For this review, take the finished solid that the model builds, in its own axes (mm). Face numbers are marked on the shaded views. Round coordinates to 2 decimals unless told otherwise and drop trailing zeros. Write each loop counter-clockwise with the first axis right and the second up, starting at its lowest first coordinate (ties: lowest second). Pieces come first, ordered by that corner, then holes. Notation, with made-up numbers: (-22, -31.75) - (-4, -31.75) arc R4 ccw to (-4, -27.75) - close; hole circle Ø2 at (-34.75, 1.25). An arc over 180 degrees is marked (long way). One line per item, written item: value. Start each with the question number.
Q1. Add section C-C on z = -231. Write out the cut boundary in (x, y), and give its area (3 significant figures).
Q2. Mouldability with a two-part tool opening along Z and no side actions: class the marked faces 1, 2 and 3 as +Z half, -Z half, draft (parallel to the pull), parting line (faces both ways), or undercut.
Q3. Add section B-B on z = -33. Write out the cut boundary in (x, y), and give its area (3 significant figures).
Q4. Clearance check with flat-ended pins moving along their axes: pin 1 Ø20.5 at (x, y) = (578.5, -461.5) entering from -Z; pin 2 Ø12.5 at (x, z) = (222, -82) entering from +Y; pin 3 Ø1 at (y, z) = (-207, -108) entering from +X. State where each tip first meets the part, or that it passes through.
Q5. Add section D-D on x = 97.5. Write out the cut boundary in (y, z).
Q6. Add section A-A on y = -127. Write out the cut boundary in (x, z), and give its area (3 significant figures).
Q7. For probe 1 along X at (y, z) = (-132.5, -85); probe 2 along Z at (x, y) = (92, -295.5); probe 3 along Z at (x, y) = (464, -364), list the stretches that pass through material, from the lowest coordinate up.
```python
from build123d import *

# Parameters (mm, degrees)
CROQUIS1_W               = 491.3875
CROQUIS1_H               = 491.3875
CROQUIS1_W_2             = 440.5875
CROQUIS1_H_2             = 440.5875
SALIENTE_EXTRUIR1_DEPTH  = 25.4
CROQUIS2_W               = 25.4
CROQUIS2_H               = 25.4
SALIENTE_EXTRUIR2_DEPTH  = 422.312858808
CROQUIS3_W               = 25.4
CROQUIS3_H               = 25.4
SALIENTE_EXTRUIR3_DEPTH  = 25.4
SALIENTE_EXTRUIR4_REACH  = 813.249
CROQUIS4_W               = 25.4
CROQUIS4_H               = 25.4
CROQUIS5_W               = 25.4
CROQUIS5_H               = 25.4
SALIENTE_EXTRUIR5_DEPTH  = 292
SALIENTE_EXTRUIR7_REACH  = 813.249
CROQUIS7_W               = 25.4
CROQUIS7_H               = 25.4
SALIENTE_EXTRUIR9_DEPTH  = 25.4
SALIENTE_EXTRUIR10_DEPTH = 25.4
SALIENTE_EXTRUIR11_REACH = 950.384
CROQUIS11_W              = 25.4
CROQUIS11_H              = 25.4
SALIENTE_EXTRUIR12_DEPTH = 25.4
SALIENTE_EXTRUIR13_REACH = 932.183
CROQUIS13_W              = 25.087212933
CROQUIS13_H              = 25.4
SALIENTE_EXTRUIR8_DEPTH  = 0.79375


with BuildPart() as part:
    # Croquis1 → Saliente-Extruir1 (new body)
    with BuildSketch(Plane(origin=(0, 0, 0), x_dir=(1, 0, 0), z_dir=(0, 1, 0))):
        with Locations((220.29375, 220.29375)):
            Rectangle(CROQUIS1_W, CROQUIS1_H)
        with Locations((220.29375, 220.29375)):
            Rectangle(CROQUIS1_W_2, CROQUIS1_H_2, mode=Mode.SUBTRACT)
    extrude(amount=-SALIENTE_EXTRUIR1_DEPTH)

    # Croquis2 → Saliente-Extruir2 (add)
    with BuildSketch(Plane.XZ.offset(25.4)):
        with Locations((453.2875, -369.3875)):
            Rectangle(CROQUIS2_W, CROQUIS2_H)
        with Locations((-12.7, -369.3875)):
            Rectangle(CROQUIS2_W, CROQUIS2_H)
    extrude(amount=SALIENTE_EXTRUIR2_DEPTH)

    # Croquis3 → Saliente-Extruir3 (add)
    with BuildSketch(Plane.XZ.offset(447.712858808)):
        with Locations((-12.7, -369.3875)):
            Rectangle(CROQUIS3_W, CROQUIS3_H)
        with Locations((453.2875, -369.3875)):
            Rectangle(CROQUIS3_W, CROQUIS3_H)
    extrude(amount=SALIENTE_EXTRUIR3_DEPTH)

    # Croquis4 → Saliente-Extruir4 (add, up to next)
    with BuildSketch(Plane(origin=(0, 0, 0), x_dir=(0, 0, -1), z_dir=(1, 0, 0)), mode=Mode.PRIVATE) as saliente_extruir4_sk1:
        with Locations((369.3875, -460.412858808)):
            Rectangle(CROQUIS4_W, CROQUIS4_H)
    saliente_extruir4_tool1 = extrude(saliente_extruir4_sk1.sketch, amount=SALIENTE_EXTRUIR4_REACH, mode=Mode.PRIVATE) - part.part
    add(saliente_extruir4_tool1.solids().sort_by_distance((0, -460.412859, -369.3875))[0])

    # Croquis5 → Saliente-Extruir5 (add)
    with BuildSketch(Plane.XY.offset(-356.6875)):
        with Locations((-12.7, -460.412858808)):
            Rectangle(CROQUIS5_W, CROQUIS5_H)
        with Locations((453.2875, -460.412858808)):
            Rectangle(CROQUIS5_W, CROQUIS5_H)
    extrude(amount=SALIENTE_EXTRUIR5_DEPTH)

    # Croquis7 → Saliente-Extruir7 (add, up to next)
    with BuildSketch(Plane(origin=(0, 0, 0), x_dir=(0, 0, -1), z_dir=(1, 0, 0)), mode=Mode.PRIVATE) as saliente_extruir7_sk1:
        with Locations((369.3875, -255.012858808)):
            Rectangle(CROQUIS7_W, CROQUIS7_H)
    saliente_extruir7_tool1 = extrude(saliente_extruir7_sk1.sketch, amount=SALIENTE_EXTRUIR7_REACH, mode=Mode.PRIVATE) - part.part
    add(saliente_extruir7_tool1.solids().sort_by_distance((0, -255.012859, -369.3875))[0])

    # Croquis9 → Saliente-Extruir9 (add)
    with BuildSketch(Plane(origin=(0, -447.712858808, 0), x_dir=(1, 0, 0), z_dir=(0, 1, 0))):
        Polygon((465.9875, 382.0875), (694.147848124, 382.0875), (694.147848124, 65.242422269), (465.9875, 65.242422269), (0, 65.242422269), (0, 90.642422269), (465.9875, 90.642422269), (668.747848124, 90.642422269), (668.747848124, 356.6875), (465.9875, 356.6875), align=None)
    extrude(amount=-SALIENTE_EXTRUIR9_DEPTH)

    # Croquis10 → Saliente-Extruir10 (add)
    with BuildSketch(Plane.XY.offset(-356.6875)):
        Polygon((668.747848124, -447.712858808), (668.747848124, -267.712858808), (465.9875, -267.712858808), (465.9875, -191.947517804), (694.147848124, -242.312858808), (694.147848124, -447.712858808), align=None)
    extrude(amount=-SALIENTE_EXTRUIR10_DEPTH)

    # Croquis11 → Saliente-Extruir11 (add, up to next)
    with BuildSketch(Plane(origin=(0, -447.712858808, 0), x_dir=(1, 0, 0), z_dir=(0, 1, 0)), mode=Mode.PRIVATE) as saliente_extruir11_sk1:
        with Locations((-12.7, 77.942422269)):
            Rectangle(CROQUIS11_W, CROQUIS11_H)
    saliente_extruir11_tool1 = extrude(saliente_extruir11_sk1.sketch, amount=SALIENTE_EXTRUIR11_REACH, mode=Mode.PRIVATE) - part.part
    # Croquis11 → Saliente-Extruir11 (add, up to next)
    with BuildSketch(Plane(origin=(0, -447.712858808, 0), x_dir=(1, 0, 0), z_dir=(0, 1, 0)), mode=Mode.PRIVATE) as saliente_extruir11_sk2:
        with Locations((453.2875, 77.942422269)):
            Rectangle(CROQUIS11_W, CROQUIS11_H)
    saliente_extruir11_tool2 = extrude(saliente_extruir11_sk2.sketch, amount=SALIENTE_EXTRUIR11_REACH, mode=Mode.PRIVATE) - part.part
    add(saliente_extruir11_tool1.solids().sort_by_distance((-12.7, -447.712859, -77.942422))[0])
    add(saliente_extruir11_tool2.solids().sort_by_distance((453.2875, -447.712859, -77.942422))[0])

    # Croquis12 → Saliente-Extruir12 (add)
    with BuildSketch(Plane(origin=(-18.750939814, -84.943750412, 0), x_dir=(0.9764914853588178, -0.21555597653911102, 0), z_dir=(0.21555597653911102, 0.9764914853588178, 0))):
        Polygon((670.444567301, 356.6875), (670.444567301, 166.558874098), (496.408260678, 166.558874098), (496.408260678, 356.6875), (441.473637421, 356.6875), (441.473637421, 90.098891747), (496.408260678, 90.098891747), (496.408260678, 141.262403959), (670.444567301, 141.262403959), (670.444567301, 64.950724727), (695.531780234, 64.950724727), (695.531780234, 356.6875), align=None)
    extrude(amount=-SALIENTE_EXTRUIR12_DEPTH)

    # Saliente-Extruir13: up to this plane
    saliente_extruir13_end = Plane(origin=(0, -447.712858808, -64.6875), z_dir=(0, -1, 0))
    # Croquis13 → Saliente-Extruir13 (add, up to the surface)
    with BuildSketch(Plane(origin=(-24.226061618, -109.74663414, 0), x_dir=(0.9764914853588177, -0.21555597653911182, 0), z_dir=(-0.21555597653911182, -0.9764914853588177, 0)), mode=Mode.PRIVATE) as saliente_extruir13_sk1:
        with Locations((682.988173768, -77.650724727)):
            Rectangle(CROQUIS13_W, CROQUIS13_H)
    saliente_extruir13_tool1 = split(extrude(saliente_extruir13_sk1.sketch, amount=SALIENTE_EXTRUIR13_REACH, mode=Mode.PRIVATE), bisect_by=saliente_extruir13_end, keep=Keep.BOTH, mode=Mode.PRIVATE)
    add(saliente_extruir13_tool1.solids().sort_by_distance((642.706075, -256.968817, -77.650725))[0])

    # Croquis8 → Saliente-Extruir8 (add)
    with BuildSketch(Plane(origin=(0, 0, -382.0875), x_dir=(-1, 0, 0), z_dir=(0, 0, -1))):
        Polygon((-465.9875, -473.112858808), (25.4, -473.112858808), (25.4, -242.312858808), (-465.9875, -242.312858808), (-694.147848124, -242.312858808), (-694.147848124, -473.112858808), align=None)
    extrude(amount=SALIENTE_EXTRUIR8_DEPTH)


solid = part.part
```
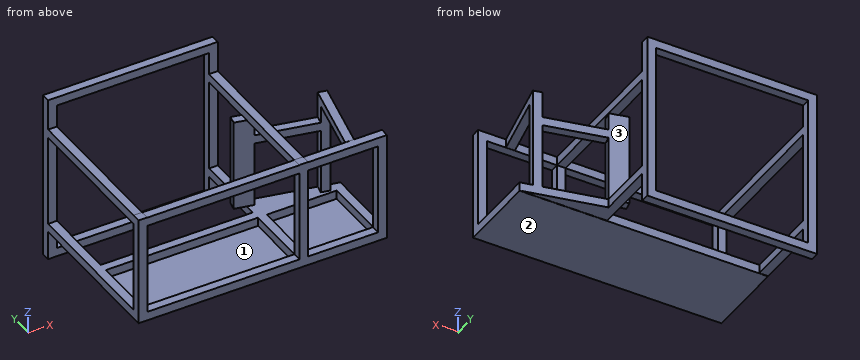
Result set:
1. outline: (-25.4, -473.11) - (0, -473.11) - (0, -447.71) - (-25.4, -447.71) - close; (-25.4, -25.4) - (0, -25.4) - (0, 0) - (-25.4, 0) - close; (406.87, -204.91) - (460.51, -216.75) - (465.99, -191.95) - (412.34, -180.11) - close; (440.59, -473.11) - (465.99, -473.11) - (465.99, -447.71) - (440.59, -447.71) - close; (440.59, -25.4) - (465.99, -25.4) - (465.99, 0) - (440.59, 0) - close; (630.46, -254.26) - (654.95, -259.67) - (660.43, -234.87) - (635.93, -229.46) - close; (668.75, -473.11) - (694.15, -473.11) - (694.15, -447.71) - (668.75, -447.71) - close
1. area: 5,260 mm^2
2. face 1: +Z half
2. face 2: -Z half
2. face 3: undercut
3. outline: (-25.4, -25.4) - (0, -25.4) - (0, 0) - (-25.4, 0) - close; (440.59, -25.4) - (465.99, -25.4) - (465.99, 0) - (440.59, 0) - close
3. area: 1,290 mm^2
4. pin 1: stops at z = -382.88
4. pin 2: stops at y = -447.71
4. pin 3: stops at x = 462.78
5. outline: (-473.11, -382.88) - (-242.31, -382.88) - (-242.31, -356.69) - (-267.71, -356.69) - (-267.71, -382.09) - (-447.71, -382.09) - (-447.71, -356.69) - (-473.11, -356.69) - close; (-473.11, -90.64) - (-447.71, -90.64) - (-447.71, -65.24) - (-473.11, -65.24) - close; (-25.4, -465.99) - (0, -465.99) - (0, -440.59) - (-25.4, -440.59) - close; (-25.4, 0) - (0, 0) - (0, 25.4) - (-25.4, 25.4) - close
6. outline: (-25.4, -382.09) - (0, -382.09) - (0, -356.69) - (-25.4, -356.69) - close; (-25.4, -90.64) - (0, -90.64) - (0, -65.24) - (-25.4, -65.24) - close; (440.59, -382.09) - (465.99, -382.09) - (465.99, -356.69) - (440.59, -356.69) - close; (440.59, -90.64) - (465.99, -90.64) - (465.99, -65.24) - (440.59, -65.24) - close
6. area: 2,580 mm^2
7. probe 1: x = -25.4 to 0, 440.59 to 465.99
7. probe 2: z = -382.88 to -382.09
7. probe 3: z = -382.88 to -356.69, -90.64 to -65.24
